Source: CAD feature listing. Evaluate the final solid. Frame: model axes, mm. Face numbers are marked on the shaded views. A direction names the side the tool comes from. Give positions to 0.01 mm unless a question says otherwise; leave off trailing zeros. Write each loop counter-clockwise with the first axis right and the second up, starting at its lowest first coordinate (ties: lowest second). Pieces come first, ordered by that corner, then holes. Notation, with made-up numbers: (-13.75, 45) - (5.25, 45) arc R5 cw to (5.25, 53) - close; hole circle Ø7 at (48.25, 5). An arc over 180 degrees is marked (long way). Answer as a JSON object with one key per item and string values. Group by question number.
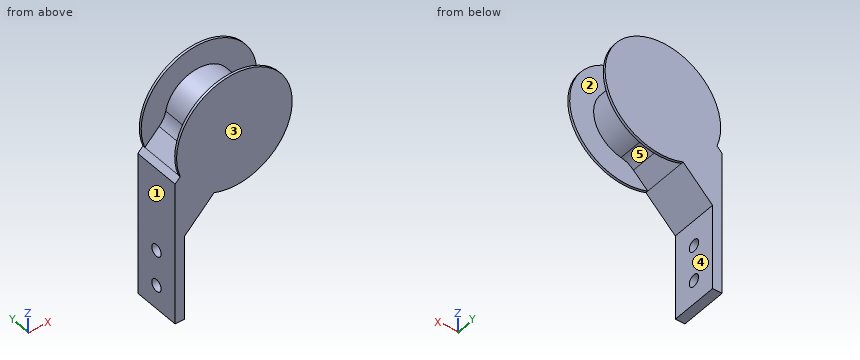
from build123d import *

# Parameters (mm, degrees)
F1_DEPTH      = 12.7
F1_DEPTH_BACK = 12.7
F2_DEPTH      = 11.43
F2_DEPTH_BACK = 11.43
F3_W          = 25.4
F3_H          = 76.2
F4_DEPTH      = 5.08
F6_D          = 6.35


with BuildPart() as f1:
    # F0 (on Front) → F1 (new body, two sides)
    with BuildSketch(Plane.XZ) as f1_sk:
        with BuildLine():
            Line((0, 17.9605122421), (0, -17.9605122421))
            Line((0, -17.9605122421), (20.6782230746, 2.7177108325))
            Line((20.6782230746, 2.7177108325), (28.2681090435, 10.3075968013))
            ThreePointArc((28.2681090435, 10.3075968013), (31.2921928816, 12.5440252054), (34.8386907134, 13.7966417449))
            ThreePointArc((34.8386907134, 13.7966417449), (44.1308964237, 44.1308964237), (13.7966417449, 34.8386907134))
            ThreePointArc((13.7966417449, 34.8386907134), (12.5440252054, 31.2921928816), (10.3075968013, 28.2681090435))
            Line((10.3075968013, 28.2681090435), (2.7177108325, 20.6782230746))
            Line((2.7177108325, 20.6782230746), (0, 17.9605122421))
        make_face()
        with BuildLine():
            Line((28.2681090435, 10.3075968013), (20.6782230746, 2.7177108325))
            ThreePointArc((20.6782230746, 2.7177108325), (53.1111525448, 53.1111525448), (2.7177108325, 20.6782230746))
            Line((2.7177108325, 20.6782230746), (10.3075968013, 28.2681090435))
            ThreePointArc((10.3075968013, 28.2681090435), (12.5440252054, 31.2921928816), (13.7966417449, 34.8386907134))
            ThreePointArc((13.7966417449, 34.8386907134), (44.1308964237, 44.1308964237), (34.8386907134, 13.7966417449))
            ThreePointArc((34.8386907134, 13.7966417449), (31.2921928816, 12.5440252054), (28.2681090435, 10.3075968013))
        make_face()
    extrude(amount=F1_DEPTH)
    extrude(f1_sk.sketch, amount=-F1_DEPTH_BACK)

    # F0 (on Front) → F2 (cut, two sides)
    with BuildSketch(Plane.XZ) as f2_sk:
        with BuildLine():
            Line((28.2681090435, 10.3075968013), (20.6782230746, 2.7177108325))
            ThreePointArc((20.6782230746, 2.7177108325), (53.1111525448, 53.1111525448), (2.7177108325, 20.6782230746))
            Line((2.7177108325, 20.6782230746), (10.3075968013, 28.2681090435))
            ThreePointArc((10.3075968013, 28.2681090435), (12.5440252054, 31.2921928816), (13.7966417449, 34.8386907134))
            ThreePointArc((13.7966417449, 34.8386907134), (44.1308964237, 44.1308964237), (34.8386907134, 13.7966417449))
            ThreePointArc((34.8386907134, 13.7966417449), (31.2921928816, 12.5440252054), (28.2681090435, 10.3075968013))
        make_face()
    extrude(amount=-F2_DEPTH, mode=Mode.SUBTRACT)
    extrude(f2_sk.sketch, amount=F2_DEPTH_BACK, mode=Mode.SUBTRACT)

    # F3 (on Right) → F4 (join)
    with BuildSketch(Plane.YZ):
        with Locations((0, -20.1394877579)):
            Rectangle(F3_W, F3_H)
    extrude(amount=F4_DEPTH)

    # F6 (through all)
    with Locations(Plane.YZ.offset(5.08)):
        with Locations((0, -26.4894877579), (0, -45.5394877579)):
            Hole(F6_D / 2)


solid = f1.part
Q1. Ray query, probe 1 along Y at (x, z) = (42, 56.5); probe 2 along Z at (x, y) = (1.05, 0); probe 3 along Z at (x, y) = (1.8, 0). Return the intervals inside material, ascending. Write a range as [from, to].
Q2. Section D-D on x = 26. Return the cut outline in (y, z).
Q3. Section A-A on y = 0. Return the cut outline in (x, z).
Q4. Reachability of the marked faces 1 and 2 from +Z, -Z, +X, -X, +Y, -Y: full face, straight path, thin tool, end or side. Return the list, or none.
Q5. Section B-B on z = 53.5. Return the cut outline in (x, y), then the cut area to 3 significant figures.
Q6. Section C-C on y = 9.5. Return the cut outline in (x, z).
Q7. Draft query along Y for the marked faces 3, 4 and 5. Return one class per face: released by +Y, released by -Y, zero draft, split by the parting line, or undercut.
Q8. First-contact query: pin 1 Ø7.5 at (y, z) = (-2.5, -29) entering from +X; pin 2 Ø1.5 at (y, z) = (-8.5, 3) entering from -X; pin 3 Ø4 at (y, z) = (-3, 6.5) entering from +X; pin 4 Ø10 at (x, y) = (42.5, 9.5) entering from -Z. Flat tips, straight axial feed; report the tip coordinate or a pass-through.
Taken from the geometry:
{
 "1": {"probe 1": "y = [-12.7, -11.43], [11.43, 12.7]", "probe 2": "z = [-58.24, -48.71], [-42.36, -29.66], [-23.31, 19.01]", "probe 3": "z = [-58.24, -48.71], [-42.36, -29.66], [-23.31, 19.76]"},
 "2": {"outline": "(-12.7, 1.26) - (-11.43, 1.26) - (-11.43, 8.04) - (11.43, 8.04) - (11.43, 1.26) - (12.7, 1.26) - (12.7, 61.61) - (11.43, 61.61) - (11.43, 48.55) - (-11.43, 48.55) - (-11.43, 61.61) - (-12.7, 61.61) - close"},
 "3": {"outline": "(0, -58.24) - (5.08, -58.24) - (5.08, -48.71) - (0, -48.71) - close; (0, -42.36) - (5.08, -42.36) - (5.08, -29.66) - (0, -29.66) - close; (0, -23.31) - (5.08, -23.31) - (5.08, -12.88) - (28.27, 10.31) arc R12.7 cw to (34.84, 13.8) arc R17.96 ccw (long way) to (13.8, 34.84) arc R12.7 cw to (10.31, 28.27) - (0, 17.96) - close"},
 "4": {"face 1": "+Z, -Z, -X, +Y, -Y", "face 2": "none"},
 "5": {"outline": "(10.15, -12.7) - (52.72, -12.7) - (52.72, -11.43) - (10.15, -11.43) - close; (10.15, 11.43) - (52.72, 11.43) - (52.72, 12.7) - (10.15, 12.7) - close", "area": "108 mm²"},
 "6": {"outline": "(0, -58.24) - (5.08, -58.24) - (5.08, -12.88) - (28.27, 10.31) arc R12.7 cw to (34.84, 13.8) arc R17.96 ccw (long way) to (13.8, 34.84) arc R12.7 cw to (10.31, 28.27) - (0, 17.96) - close"},
 "7": {"face 3": "released by -Y", "face 4": "zero draft", "face 5": "undercut"},
 "8": {"pin 1": "stops at x = 5.08", "pin 2": "stops at x = 0", "pin 3": "stops at x = 26.46", "pin 4": "stops at z = 1.46"}
}
